Solid Edge part; units mm, degrees
sketch "Sketch1" plane through (0, 0, 0) normal (0, 0, -1) x (-1, 0, 0)
  circle A0 centre (0, 0) radius 2
  circle A1 centre (0, 0) radius 3.495
extrude "Protrusion1" add sketch "Sketch1" along normal blind 30
sketch "Sketch2" plane through (0, 0, 0) normal (0, -1, 0) x (1, 0, 0)
  line L0 (-7.0834, -20) -> (-7.0834, -5)
  line L1 (-7.0834, -5) -> (-3, -5)
  line L2 (-3, -5) -> (-3, -20)
  line L3 (-3, -20) -> (-7.0834, -20)
  arc A0 (-3.495, -4.7834) -> (-2.2003, 1.0477) centre (10.2833, -4.7834) cw
  line L4 (-2.2003, 1.0477) -> (-7.5454, 0.1871)
  line L5 (-7.5454, 0.1871) -> (-7.0698, -4.6128)
  line L6 (-7.0698, -4.6128) -> (-3.495, -4.7834)
revolve "RevolvedCutout1" cut sketch "Sketch2" angle 360 about axis through (0, 0, 0) along (0, 0, 1)
properties material "Réz, sárgaréz"
Check sheet for the modelled part. Datum: model origin and axes. Units: mm. A direction names the side the tool comes from. Give positions to 0.01 mm unless a question says otherwise; leave off trailing zeros. Write each loop counter-clockwise with the first axis right and the second up, starting at its lowest first coordinate (ties: lowest second). Pieces come first, ordered by that corner, then holes.
Item 1: Cross-section at B-B (z = -6.5). Enter the section's corners in (x, y).
Item 2: Access from +Z, -Z, +X, -X, +Y, -Y to the whole of each face (thin tool, end or side, straight path). Record for faces 4 (the face through (-1, -3, -20)), 5 (the face through (-1, 2, 0)).
Item 3: Scan lines: L1, parallel to Y at x = 0, z = -12; L2, parallel to Y at x = 0, z = -21.75 (3 decimals); L3, parallel to X at y = -1.5, z = -17.5. Record each from-to range of solid material in increasing order.
Item 4: Gauge pin test, flat ends, axial feed: pin 1 (4 mm diameter, centred on y = -2.5, z = -9.5, fed in from +X); pin 2 (3.5 mm diameter, centred on x = 0.5, y = 1, fed in from -Z); pin 3 (1.5 mm diameter, centred on y = 0.5, z = -6, fed in from -X); pin 4 (1 mm diameter, centred on x = 1.5, z = -17.5, fed in from +Y). Record the tip position at first contact, or that the pin passes through.
Item 5: Draft check along Z on faces 1 (the face through (-2, -2, -30)), 2 (the face through (-1, -3, -5)), 3 (the face through (0.76, 3.41, -24.93)). Enter one of: released by +Z, released by -Z, zero draft, split by the parting line, or undercut.
Item 6: Cross-section at A-A (z = -26). Enter the section's corners in (x, y) (3 decimals), and give its area (3 significant figures).
Report:
1. outline: circle Ø6 at (0, 0); hole circle Ø4 at (0, 0)
2. face 4: none
2. face 5: +Z, +X, -X, +Y, -Y
3. L1: y = -3 to -2, 2 to 3
3. L2: y = -3.495 to -2, 2 to 3.495
3. L3: x = -2.6 to -1.32, 1.32 to 2.6
4. pin 1: stops at x = 2.96
4. pin 2: stops at z = -30
4. pin 3: stops at x = -3
4. pin 4: stops at y = 2.83
5. face 1: released by -Z
5. face 2: undercut
5. face 3: zero draft
6. outline: circle Ø6.99 at (0, 0); hole circle Ø4 at (0, 0)
6. area: 25.8 mm2
